Check sheet for the drawn part. Datum: minimum x, y, z corner. Units: mm. A direction names the side the tool comes from. Coordinates: 2 decimals unless noted, no trailing zeros. Loops run counter-clockwise (first coordinate to the right, second up) from the corner with the lowest first, then second, coordinate; pieces in that order, holes last.
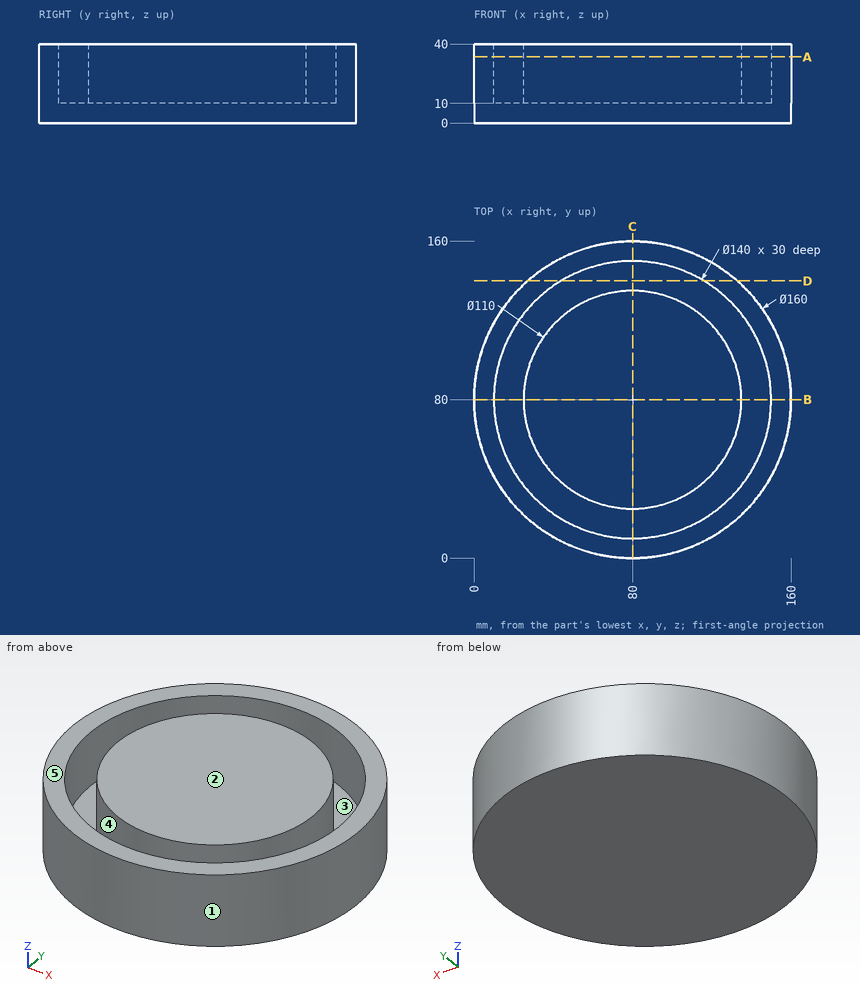
(1) Sectioned sample at D-D on y = 140. Record the cut outline in (x, z), and give its area (3 significant figures).
Findings:
outline: (27.08, 0) - (132.92, 0) - (132.92, 40) - (116.06, 40) - (116.06, 10) - (43.94, 10) - (43.94, 40) - (27.08, 40) - close
area: 2,070 mm2
(2) Draft check along Y on the marked faces 1, 2 and 3. Enter one of: +Y half, -Y half, draft (parallel to the pull), parting line (faces both ways), or undercut.
Findings:
face 1: parting line
face 2: draft
face 3: undercut
(3) Gauge pin test, flat ends, axial feed: pin 1 Ø5 at (x, z) = (143.5, 31) entering from -Y; pin 2 Ø8 at (y, z) = (49, 21.5) entering from +X; pin 3 Ø5 at (y, z) = (113, 30.5) entering from +X. Record the tip position at first contact, or that the pin passes through.
Findings:
pin 1: stops at y = 28.24
pin 2: stops at x = 155.31
pin 3: stops at x = 153.96
(4) Scan lines: L1, parallel to Y at x = 80, z = 30; L2, parallel to Y at x = 55.5, z = 18.5; L3, parallel to X at y = 115, z = 38. Record each from-to range of solid material in increasing order.
Findings:
L1: y = 0 to 10, 25 to 135, 150 to 160
L2: y = 3.84 to 14.43, 30.76 to 129.24, 145.57 to 156.16
L3: x = 8.06 to 19.38, 37.57 to 122.43, 140.62 to 151.94
(5) Access from +Z, -Z, +X, -X, +Y, -Y to the whole of each face (thin tool, end or side, straight path). Record for the marked faces 4 and 5.
Findings:
face 4: +Z
face 5: +Z, +X, -X, +Y, -Y
(6) Sectioned sample at A-A on z = 33.5. Record the cut outline in (x, y).
Findings:
outline: circle Ø160 at (80, 80); circle Ø110 at (80, 80); hole circle Ø140 at (80, 80)
(7) Sectioned sample at B-B on y = 80. Record the cut outline in (x, z), and give its area (3 significant figures).
Findings:
outline: (0, 0) - (160, 0) - (160, 40) - (150, 40) - (150, 10) - (135, 10) - (135, 40) - (25, 40) - (25, 10) - (10, 10) - (10, 40) - (0, 40) - close
area: 5,500 mm2
